The model under review builds one solid part; all positions refer to its coordinate system, in mm. A direction names the side the tool comes from. Coordinates: 2 decimals unless noted, no trailing zeros. Write each loop counter-clockwise with the first axis right and the second up, starting at its lowest first coordinate (ties: lowest second). Pieces come first, ordered by that corner, then holes.
1) For P1, Ø0.8, axis at y = 2, z = -12, coming from the -X side; P2, Ø5, axis at x = 15.25, z = -15.25, coming from the -Y side; P3, Ø2, axis at x = -10, z = -13, coming from the +Y side; P4, Ø2.5, axis at x = 15.25, z = 15.25, coming from the -Y side, all flat-tipped, find the tip position at first contact; note any pin that passes through.
2) Machinability: for faces 1 (the flat face through (-17, 3, -1)), 2 (the flat face through (-5, 2, -10)), 3 (the flat face through (-17, 3, -9)), 4 (the flat face through (12, 3, 0)), 5 (the flat face through (-5, 2, 5)), which of the approach directions +Z, -Z, +X, -X, +Y, -Y give a long, thin tool a straight path to every point of the face, cutting with its end or side? Answer none if there is none.
3) For line 1 (Z direction, x = 15.25, y = 1.25); line 2 (X direction, y = 1.55, z = -4.5), list the stretches that pass through material, from the lowest coordinate up.
4) Add section D-D, the plane x = -9. State the section outline as (y, z) points.
5) Add section C-C, the plane y = 0.95. State the section outline as (x, z) points.
6) Add section B-B, the plane x = -15.25. State the section outline as (y, z) points.
7) Mouldability with a two-part tool opening along Z and no side actions: class faces 6 (the flat face through (-5, 3, 0)), 7 (the cylindrical face through (15.18, 0.74, -13.75)), 8 (the flat face through (-5, 2, -5)), 9 (the flat face through (18.507, 0.74, -18.457)) as released by +Z, released by -Z, zero draft, split by the parting line, or undercut.
8) Add section A-A, the plane z = -15.25. State the section outline as (x, y) points.
from build123d import *

# Parameters (mm, degrees)
SKETCH1_R           = 1.5
BOSS_EXTRUDE1_DEPTH = 1.5
SKETCH2_W           = 10
SKETCH2_H           = 10
SKETCH2_W_2         = 5
SKETCH2_W_3         = 3
SKETCH2_H_2         = 3
BOSS_EXTRUDE2_DEPTH = 1.5
SKETCH3_W           = 6
SKETCH3_H           = 8
BOSS_EXTRUDE3_DEPTH = 3


with BuildPart() as part:
    # Sketch1 → Boss-Extrude1 (new body)
    with BuildSketch(Plane(origin=(0, 0, 0), x_dir=(1, 0, 0), z_dir=(0, 1, 0))):
        Polygon((16.714466094, 20.25), (-16.714466094, 20.25), (-20.25, 16.714466094), (-20.25, -16.714466094), (-16.714466094, -20.25), (16.714466094, -20.25), (20.25, -16.714466094), (20.25, 16.714466094), align=None)
        with Locations(Location((-15.25, 15.25, 0), (0, 0, 270))):
            Circle(SKETCH1_R, mode=Mode.SUBTRACT)
        with Locations(Location((-15.25, -15.25, 0), (0, 0, 270))):
            Circle(SKETCH1_R, mode=Mode.SUBTRACT)
        with Locations(Location((15.25, -15.25, 0), (0, 0, 90))):
            Circle(SKETCH1_R, mode=Mode.SUBTRACT)
        with Locations(Location((15.25, 15.25, 0), (0, 0, 90))):
            Circle(SKETCH1_R, mode=Mode.SUBTRACT)
    extrude(amount=BOSS_EXTRUDE1_DEPTH)

    # Sketch2 → Boss-Extrude2 (add)
    with BuildSketch(Plane(origin=(0, 1.5, 0), x_dir=(1, 0, 0), z_dir=(0, 1, 0))):
        with Locations((-5, 0)):
            Rectangle(SKETCH2_W, SKETCH2_H)
        with Locations((12.5, 0)):
            Rectangle(SKETCH2_W_2, SKETCH2_H)
        with Locations((-5, 11.5)):
            Rectangle(SKETCH2_W_3, SKETCH2_H_2)
    extrude(amount=BOSS_EXTRUDE2_DEPTH)

    # Sketch3 → Boss-Extrude3 (add)
    with BuildSketch(Plane(origin=(0, 1.5, 0), x_dir=(1, 0, 0), z_dir=(0, 1, 0))):
        with Locations((-17.25, 5)):
            Rectangle(SKETCH3_W, SKETCH3_H)
    extrude(amount=BOSS_EXTRUDE3_DEPTH)


solid = part.part
Geometry results:
1. P1: stops at x = -6.5
1. P2: stops at y = 0
1. P3: stops at y = 1.5
1. P4: passes through
2. face 1: +Z, -X, +Y
2. face 2: +X, -X, +Y
2. face 3: -Z, +X, -X, +Y
2. face 4: +Z, -Z, +X, +Y
2. face 5: +Z, +X, -X, +Y
3. line 1: z = -20.25 to -16.75, -13.75 to 13.75, 16.75 to 20.25
3. line 2: x = -20.25 to -14.25, -10 to 0, 10 to 15
4. outline: (0, -20.25) - (1.5, -20.25) - (1.5, -5) - (3, -5) - (3, 5) - (1.5, 5) - (1.5, 20.25) - (0, 20.25) - close
5. outline: (-20.25, -16.71) - (-16.71, -20.25) - (16.71, -20.25) - (20.25, -16.71) - (20.25, 16.71) - (16.71, 20.25) - (-16.71, 20.25) - (-20.25, 16.71) - close; hole circle Ø3 at (-15.25, -15.25); hole circle Ø3 at (-15.25, 15.25); hole circle Ø3 at (15.25, -15.25); hole circle Ø3 at (15.25, 15.25)
6. outline: (0, -20.25) - (1.5, -20.25) - (1.5, -16.75) - (0, -16.75) - close; (0, -13.75) - (1.5, -13.75) - (1.5, -9) - (4.5, -9) - (4.5, -1) - (1.5, -1) - (1.5, 13.75) - (0, 13.75) - close; (0, 16.75) - (1.5, 16.75) - (1.5, 20.25) - (0, 20.25) - close
7. face 6: zero draft
7. face 7: undercut
7. face 8: undercut
7. face 9: released by -Z
8. outline: (-20.25, 0) - (-16.75, 0) - (-16.75, 1.5) - (-20.25, 1.5) - close; (-13.75, 0) - (13.75, 0) - (13.75, 1.5) - (-13.75, 1.5) - close; (16.75, 0) - (20.25, 0) - (20.25, 1.5) - (16.75, 1.5) - close
